For this review, take the finished solid that the model builds, in its own axes (mm). Face numbers are marked on the shaded views. A direction names the side the tool comes from. Coordinates: 2 decimals unless noted, no trailing zeros. Loops run counter-clockwise (first coordinate to the right, second up) from the corner with the lowest first, then second, coordinate; pieces in that order, holes last.
1. Take a section at B-B, the plane y = 9.75. State the section outline as (x, z) points, then the cut area to 3 significant figures.
2. Mouldability with a two-part tool opening along X and no side actions: class the marked faces 1, 2 and 3 as pulls with the +X half, pulls with the -X half, needs draft (parallel to the pull), parting line crosses it, or undercut.
3. Machinability: for the marked faces 4, 5, 6 and 7, which of the approach directions +Z, -Z, +X, -X, +Y, -Y give a long, thin tool a straight path to every point of the face, cutting with its end or side? Answer none if there is none.
4. Take a section at C-C, the plane x = 12.75. State the section outline as (y, z) points, then the cut area to 3 significant figures.
5. Take a section at A-A, the plane x = -15.75. State the section outline as (y, z) points, then the cut area to 3 significant figures.
6. Clearance check with flat-ended pins moving along their axes: P1, Ø12, axis at x = 2.5, y = 1.5, coming from the +Z side; P2, Ø3, axis at y = 8.5, z = 6.5, coming from the -X side; P3, Ø1.7, axis at x = -15.5, y = 1.5, coming from the +Z side; P4, Ø2.5, axis at x = -8.5, y = 9, coming from the -Z side. State where each tip first meets the part, or that it passes through.
7. To check wall thickness, follow probe 1 along Y at (x, z) = (13.65, 0.4); probe 2 along Z at (x, y) = (-7, 6.75); probe 3 along Y at (x, z) = (5.25, 0.5). State the ranges of each line that lie inside material, in increasing order.
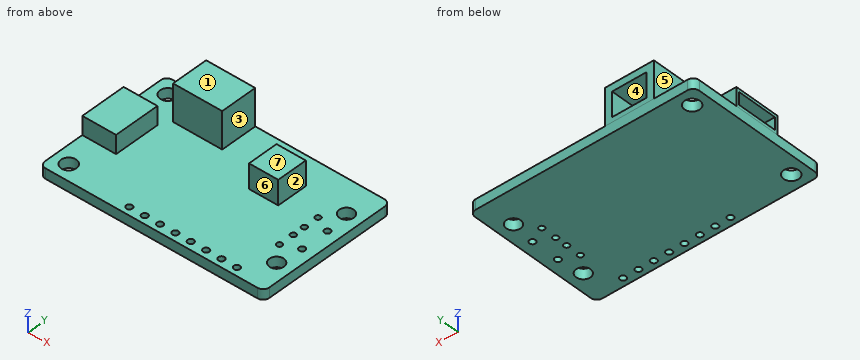
```python
from build123d import *

# Parameters (mm, degrees)
BASE_DEPTH          = 1.65
SKETCH2_R           = 1.25
CUT_EXTRUDE1_DEPTH  = 22.634116575
SKETCH3_R           = 0.5
CUT_EXTRUDE2_DEPTH  = 22.634116575
LPATTERN1_COUNT     = 8
LPATTERN1_PITCH     = 2.5
SKETCH4_R           = 1.175
CUT_EXTRUDE3_DEPTH  = 22.634116575
SKETCH9_R           = 0.45
CUT_EXTRUDE6_DEPTH  = 22.634116575
SKETCH10_R          = 0.5
CUT_EXTRUDE7_DEPTH  = 22.634116575
SKETCH5_W           = 8
SKETCH5_H           = 6
BOSS_EXTRUDE2_DEPTH = 6
SKETCH6_W           = 5.6
SKETCH6_H           = 4
CUT_EXTRUDE4_DEPTH  = 4.8
SKETCH7_W           = 5.5
SKETCH7_H           = 7.5
BOSS_EXTRUDE3_DEPTH = 3
SKETCH8_W           = 2
SKETCH8_H           = 6.5
CUT_EXTRUDE5_DEPTH  = 5
SKETCH11_W          = 4.75
SKETCH11_H          = 5
BOSS_EXTRUDE4_DEPTH = 4


with BuildPart() as part:
    # Sketch1 → Base (new body)
    with BuildSketch(Plane.XY):
        with BuildLine():
            Line((-17.25, -11.5), (17.25, -11.5))
            ThreePointArc((17.25, -11.5), (17.957106781, -11.207106781), (18.25, -10.5))
            Line((18.25, -10.5), (18.25, 10.5))
            ThreePointArc((18.25, 10.5), (17.957106781, 11.207106781), (17.25, 11.5))
            Line((17.25, 11.5), (-17.25, 11.5))
            ThreePointArc((-17.25, 11.5), (-17.957106781, 11.207106781), (-18.25, 10.5))
            Line((-18.25, 10.5), (-18.25, -10.5))
            ThreePointArc((-18.25, -10.5), (-17.957106781, -11.207106781), (-17.25, -11.5))
        make_face()
    extrude(amount=BASE_DEPTH)

    # Sketch2 → Cut-Extrude1 (cut, through all)
    with BuildSketch(Plane.XY.offset(1.65)):
        with Locations((-15.75, 9)):
            Circle(SKETCH2_R)
    cut_extrude1 = extrude(amount=-CUT_EXTRUDE1_DEPTH, mode=Mode.SUBTRACT)

    # Mirror1: Cut-Extrude1 across plane
    add(cut_extrude1.mirror(Plane.ZX), mode=Mode.SUBTRACT)

    # Sketch3 → Cut-Extrude2 (cut, through all)
    with BuildSketch(Plane.XY.offset(1.65)):
        with Locations((12.75, -10.25)):
            Circle(SKETCH3_R)
    cut_extrude2 = extrude(amount=-CUT_EXTRUDE2_DEPTH, mode=Mode.SUBTRACT)

    # LPattern1: Cut-Extrude2 ×8
    with Locations(*[(-i * LPATTERN1_PITCH, 0, 0) for i in range(1, LPATTERN1_COUNT)]):
        add(cut_extrude2, mode=Mode.SUBTRACT)

    # Sketch4 → Cut-Extrude3 (cut, through all)
    with BuildSketch(Plane.XY.offset(1.65)):
        with Locations((15.730877355, -6.3475)):
            Circle(SKETCH4_R)
    cut_extrude3 = extrude(amount=-CUT_EXTRUDE3_DEPTH, mode=Mode.SUBTRACT)

    # Sketch9 → Cut-Extrude6 (cut, through all)
    with BuildSketch(Plane.XY.offset(1.65)):
        with Locations((13.65, 1)):
            Circle(SKETCH9_R)
        with Locations((13.65, 3.5)):
            Circle(SKETCH9_R)
    cut_extrude6 = extrude(amount=-CUT_EXTRUDE6_DEPTH, mode=Mode.SUBTRACT)

    # Sketch10 → Cut-Extrude7 (cut, through all)
    with BuildSketch(Plane.XY.offset(1.65)):
        with Locations((16.25, 2.3)):
            Circle(SKETCH10_R)
    cut_extrude7 = extrude(amount=-CUT_EXTRUDE7_DEPTH, mode=Mode.SUBTRACT)

    # Mirror2: Cut-Extrude3 across plane
    add(cut_extrude3.mirror(Plane.ZX), mode=Mode.SUBTRACT)

    # Mirror3: Cut-Extrude6 across plane
    add(cut_extrude6.mirror(Plane.ZX), mode=Mode.SUBTRACT)

    # Mirror4: Cut-Extrude7 across plane
    add(cut_extrude7.mirror(Plane.ZX), mode=Mode.SUBTRACT)

    # Sketch5 → Boss-Extrude2 (add)
    with BuildSketch(Plane.XY.offset(1.65)):
        with Locations((-7.75, 8.49)):
            Rectangle(SKETCH5_W, SKETCH5_H)
    extrude(amount=BOSS_EXTRUDE2_DEPTH)

    # Sketch6 → Cut-Extrude4 (cut)
    with BuildSketch(Plane(origin=(0, 11.5, 0), x_dir=(1, 0, 0), z_dir=(0, 1, 0))):
        with Locations((-7.75, -4.45)):
            Rectangle(SKETCH6_W, SKETCH6_H)
    extrude(amount=-CUT_EXTRUDE4_DEPTH, mode=Mode.SUBTRACT)

    # Sketch7 → Boss-Extrude3 (add)
    with BuildSketch(Plane.XY.offset(1.65)):
        with Locations((-15.49, 0)):
            Rectangle(SKETCH7_W, SKETCH7_H)
    extrude(amount=BOSS_EXTRUDE3_DEPTH)

    # Sketch8 → Cut-Extrude5 (cut)
    with BuildSketch(Plane.ZY.offset(18.24)):
        with Locations((3.15, 0)):
            Rectangle(SKETCH8_W, SKETCH8_H)
    extrude(amount=-CUT_EXTRUDE5_DEPTH, mode=Mode.SUBTRACT)

    # Sketch11 → Boss-Extrude4 (add)
    with BuildSketch(Plane.XY.offset(1.65)):
        with Locations((6.125, 4.5)):
            Rectangle(SKETCH11_W, SKETCH11_H)
    extrude(amount=BOSS_EXTRUDE4_DEPTH)


solid = part.part
```
Results list:
1. outline: (-18.25, 0) - (-16.75, 0) - (-16.75, 1.65) - (-18.25, 1.65) - close; (-14.75, 0) - (18.25, 0) - (18.25, 1.65) - (-3.75, 1.65) - (-3.75, 7.65) - (-11.75, 7.65) - (-11.75, 1.65) - (-14.75, 1.65) - close; hole (-10.55, 2.45) - (-4.95, 2.45) - (-4.95, 6.45) - (-10.55, 6.45) - close
1. area: 82.5 mm2
2. face 1: needs draft
2. face 2: pulls with the +X half
2. face 3: undercut
3. face 4: +Y
3. face 5: +Z, -X, +Y, -Y
3. face 6: +Z, +X, -Y
3. face 7: +Z, +X, +Y, -Y
4. outline: (-11.5, 0) - (-10.75, 0) - (-10.75, 1.65) - (-11.5, 1.65) - close; (-9.75, 0) - (11.5, 0) - (11.5, 1.65) - (-9.75, 1.65) - close
4. area: 36.3 mm2
5. outline: (-11.5, 0) - (-10.25, 0) - (-10.25, 1.65) - (-11.5, 1.65) - close; (-7.75, 0) - (7.75, 0) - (7.75, 1.65) - (3.75, 1.65) - (3.75, 4.65) - (-3.75, 4.65) - (-3.75, 1.65) - (-7.75, 1.65) - close; (10.25, 0) - (11.5, 0) - (11.5, 1.65) - (10.25, 1.65) - close; hole (-3.25, 2.15) - (3.25, 2.15) - (3.25, 4.15) - (-3.25, 4.15) - close
5. area: 39.2 mm2
6. P1: stops at z = 5.65
6. P2: stops at x = -11.75
6. P3: stops at z = 4.65
6. P4: stops at z = 0
7. probe 1: y = -11.5 to -3.95, -3.05 to -1.45, -0.55 to 0.55, 1.45 to 3.05, 3.95 to 11.5
7. probe 2: z = 0 to 2.45, 6.45 to 7.65
7. probe 3: y = -11.5 to -10.75, -9.75 to 11.5
